```python
from build123d import *

# Parameters (mm, degrees)
SKETCH1_W           = 139.5
SKETCH1_H           = 152.4
BOSS_EXTRUDE1_DEPTH = 6.35
SKETCH2_W           = 139.5
SKETCH2_H           = 152.4
CUT_EXTRUDE1_DEPTH  = 3.375
SKETCH3_R           = 2.286
BOSS_EXTRUDE2_DEPTH = 12.7
SKETCH4_R           = 2.286
BOSS_EXTRUDE3_DEPTH = 12.7
SKETCH5_W           = 14.986
SKETCH5_H           = 13.7795
CUT_EXTRUDE2_DEPTH  = 3.975


with BuildPart() as part:
    # Sketch1 → Boss-Extrude1 (new body)
    with BuildSketch(Plane(origin=(0, 0, 0), x_dir=(1, 0, 0), z_dir=(0, 1, 0))):
        with Locations((69.75, 76.2)):
            Rectangle(SKETCH1_W, SKETCH1_H)
    extrude(amount=BOSS_EXTRUDE1_DEPTH)

    # Sketch2 → Cut-Extrude1 (cut)
    with BuildSketch(Plane(origin=(0, 6.35, 0), x_dir=(1, 0, 0), z_dir=(0, 1, 0))):
        with Locations((69.75, 76.2)):
            Rectangle(SKETCH2_W, SKETCH2_H)
    extrude(amount=-CUT_EXTRUDE1_DEPTH, mode=Mode.SUBTRACT)

    # Sketch3 → Boss-Extrude2 (add)
    with BuildSketch(Plane.XY):
        with BuildLine():
            Line((63.4, 9.325), (63.4, 2.975))
            Line((63.4, 2.975), (76.1, 2.975))
            Line((76.1, 2.975), (76.1, 9.325000158))
            ThreePointArc((76.1, 9.325000158), (69.749999921, 15.675000158), (63.4, 9.325))
        make_face()
        with Locations((69.75, 9.325000158)):
            Circle(SKETCH3_R, mode=Mode.SUBTRACT)
    extrude(amount=-BOSS_EXTRUDE2_DEPTH)

    # Sketch4 → Boss-Extrude3 (add)
    with BuildSketch(Plane(origin=(0, 0, -152.4), x_dir=(-1, 0, 0), z_dir=(0, 0, -1))):
        with BuildLine():
            Line((-130.61, 9.325), (-130.61, 2.975))
            Line((-130.61, 2.975), (-117.91, 2.975))
            Line((-117.91, 2.975), (-117.91, 9.325))
            ThreePointArc((-117.91, 9.325), (-124.26, 15.675), (-130.61, 9.325))
        make_face()
        with Locations((-124.26, 9.325)):
            Circle(SKETCH4_R, mode=Mode.SUBTRACT)
        with BuildLine():
            Line((-21.59, 9.325), (-21.59, 2.975))
            Line((-21.59, 2.975), (-8.89, 2.975))
            Line((-8.89, 2.975), (-8.89, 9.325))
            ThreePointArc((-8.89, 9.325), (-15.24, 15.675), (-21.59, 9.325))
        make_face()
        with Locations((-15.24, 9.325)):
            Circle(SKETCH4_R, mode=Mode.SUBTRACT)
    extrude(amount=-BOSS_EXTRUDE3_DEPTH)

    # Sketch5 → Cut-Extrude2 (cut, through all)
    with BuildSketch(Plane(origin=(0, 2.975, 0), x_dir=(1, 0, 0), z_dir=(0, 1, 0))):
        with Locations((29.083, 139.16025)):
            Rectangle(SKETCH5_W, SKETCH5_H)
    extrude(amount=-CUT_EXTRUDE2_DEPTH, mode=Mode.SUBTRACT)


solid = part.part
```
The model under review builds one solid part; all positions refer to its coordinate system, in mm. A direction names the side the tool comes from. Round coordinates to 2 decimals unless told otherwise and drop trailing zeros. Loops run counter-clockwise (first coordinate to the right, second up) from the corner with the lowest first, then second, coordinate; pieces in that order, holes last.
1) Consider section B-B on x = 124.26. State the section outline as (y, z) points (3 decimals).
Values follow:
outline: (0, -152.4) - (7.039, -152.4) - (7.039, -139.7) - (2.975, -139.7) - (2.975, 0) - (0, 0) - close; (11.611, -152.4) - (15.675, -152.4) - (15.675, -139.7) - (11.611, -139.7) - close
2) Tool access review of faces 5 (the face through (117.91, 6, -146)), 6 (the face through (130.61, 6, -146)), 7 (the face through (15.3, 6.6, -139.7)), 8 (the face through (8.89, 6, -146)): name each direction out of +Z, -Z, +X, -X, +Y, -Y from which nothing blocks a thin tool from reaching the whole face with its end or side.
Values follow:
face 5: +Z, -Z, +Y
face 6: +Z, -Z, +X, +Y
face 7: +Z, +X, -X, +Y
face 8: +Z, -Z, -X, +Y
3) Consider section C-C on z = -96. State the section outline as (x, y) points (3 decimals), then the cut area to 3 significant figures.
Values follow:
outline: (0, 0) - (139.5, 0) - (139.5, 2.975) - (0, 2.975) - close
area: 415 mm2
4) The part is to be moulded in two halves that separate along Z. For faces 1 (the face through (69, 4, 0)), 2 (the face through (63.4, 6, -6)), 3 (the face through (69.7, 6.6, -12.7)), 4 (the face through (21.59, 5, -142)), say which applies: pulls with the +Z half, pulls with the -Z half, needs draft (parallel to the pull), parting line crosses it, or undercut.
Values follow:
face 1: pulls with the +Z half
face 2: needs draft
face 3: pulls with the -Z half
face 4: undercut
5) Consider section A-A on y = 5.25. State the section outline as (x, z) points, then the cut area to 3 significant figures.
Values follow:
outline: (8.89, -152.4) - (21.59, -152.4) - (21.59, -139.7) - (8.89, -139.7) - close; (63.4, -12.7) - (76.1, -12.7) - (76.1, 0) - (63.4, 0) - close; (117.91, -152.4) - (130.61, -152.4) - (130.61, -139.7) - (117.91, -139.7) - close
area: 484 mm2
6) Clearance check with flat-ended pins moving along their axes: P1, Ø1, axis at x = 27, y = 4, coming from the -Z side; P2, Ø1.9, axis at y = 6, z = -145.5, coming from the -X side; P3, Ø3, axis at x = 63.5, y = 6, coming from the -Z side; P4, Ø6.5, axis at x = 124, y = 10.5, coming from the +Z side. State where each tip first meets the part, or that it passes through.
Values follow:
P1: passes through
P2: stops at x = 8.89
P3: stops at z = -12.7
P4: stops at z = -139.7
7) Wall thickness on line 1 along Y through (x, z) = (8, -76) (3 decimals); line 2 along X through (y, z) = (6, -144.5); line 3 along Y through (x, z) = (69.75, -3.75) (3 decimals): over which ranges is each line inside the solid? List them lowest first.
Values follow:
line 1: y = 0 to 2.975
line 2: x = 8.89 to 21.59, 117.91 to 130.61
line 3: y = 0 to 7.039, 11.611 to 15.675
